Input: part model. Units: mm. Frame: model coordinates. A direction names the side the tool comes from. Give positions to 0.01 mm unless a question says otherwise; leave off trailing zeros. Loops run counter-clockwise (first coordinate to the right, second up) from the corner with the lowest first, then second, coordinate; pieces in that order, holes last. Notation, with made-up numbers: M -40,-14 L -29,-14 A24 ccw -29,10 Z; hole C 6.5,60 d11. An arc over 180 degrees is marked long. Use CSV: the item, a comma, the result in double quotes. Start each with the question number.
Q1. Reachability of faces 4 (the cylindrical face through (10.994, -24.204, 18.559)), 5 (the flat face through (4, 21.5, 0)) from +Z, -Z, +X, -X, +Y, -Y: full face, straight path, thin tool, end or side. Return the list, or none.
Q2. Section C-C, the plane x = -2.5. Output: boundary loops of the cut face in (y, z).
Q3. Pin query (flat end, axial travel): pin 1 (8 mm diameter, centred on y = -35, z = -61, fed in from +X); pin 2 (8 mm diameter, centred on x = 9, z = -45, fed in from -Y); pin 3 (4 mm diameter, centred on y = 40.5, z = 16.5, fed in from -X). Return the tip coordinate at first contact, or that it passes through.
Q4. Section A-A, the plane z = 0. Output: boundary loops of the cut face in (x, y), plus the area to 3 significant figures.
Q5. Material intervals for line 1 along Z through (x, y) = (-3, 0); line 2 along X through (y, z) = (37, 78.5); line 3 along X through (y, z) = (-57, 47), sorted ascending.
Q6. Section B-B, the plane y = 0. Output: boundary loops of the cut face in (x, z).
Q7. Pull-direction query (Y, two-part tool) for faces 1 (the cylindrical face through (5.463, -17.485, 0.713)), 2 (the flat face through (-13.6, -7.4, -16.2)), 3 (the conical face through (23, 20.87, -6.57)); classes: released by +Y, released by -Y, zero draft, split by the parting line, or undercut.
Autodesk Inventor part; units mm, degrees
ref_plane "YZ Plane" through (0, 0, 0) normal (1, 0, 0) x (0, 1, 0)
ref_plane "XZ Plane" through (0, 0, 0) normal (0, 1, 0) x (-1, 0, 0)
ref_plane "XY Plane" through (0, 0, 0) normal (0, 0, 1) x (1, 0, 0)
sketch "Sketch1" plane through (0, 0, 0) normal (0, 0, 1) x (1, 0, 0)
  line L0 (0, 87.5) -> (8, 87.5)
  line L1 (24, 0) -> (24, 17.5)
  line L2 (8, 87.5) -> (24, 17.5)
  line L3 (16, 0) -> (16, 17.5)
  line L4 (16, 17.5) -> (0, 87.5)
  line L5 (16, 0) -> (24, 0)
  point P0 (0, 0)
  dimension "d0" = 87.5
  dimension "d1" = 8
  dimension "d3" = 17.5
  dimension "d7" = 8
  dimension "d8" = 167.125
  dimension "d9" = 175
  dimension "d10" = 24
revolve "Revolution1" add sketch "Sketch1" angle 360 about axis through (16, 0, 0) along (1, 0, 0)
sketch "Sketch2" plane through (0, 0, 0) normal (0, 0, 1) x (1, 0, 0)
  line L0 (16, 0) -> (16, 24.5)
  line L1 (16, -17.5) -> (16, 17.5)
  line L2 (14.4, 24.5) -> (16, 24.5)
  line L3 (14.4, 24.5) -> (-13.6, 24.5)
  line L4 (-13.6, 24.5) -> (-13.6, 0)
  line L5 (-13.6, 0) -> (16, 0)
  point P0 (0, 0)
  dimension "d13" = 24.5
  dimension "d15" = 28
revolve "Revolution2" add sketch "Sketch2" angle 360 about axis through (-13.6, 0, 0) along (1, 0, 0)
sketch "Sketch3" plane through (0, 0, 0) normal (0, 0, 1) x (1, 0, 0)
  line L0 (14.4, 0) -> (14.4, 30.5)
  line L1 (14.4, 30.5) -> (13.0159, 30.5)
  line L2 (13.0159, 30.5) -> (9.0159, 30.5)
  line L3 (9.0159, 30.5) -> (9.0159, 0)
  line L4 (9.0159, 0) -> (14.4, 0)
  point P0 (0, 0)
  dimension "d17" = 30.5
  dimension "d18" = 4
revolve "Revolution3" add sketch "Sketch3" angle 360 about axis through (9.0159, 0, 0) along (1, 0, 0)
sketch "Sketch4" plane through (24, 0, 0) normal (1, 0, 0) x (0, 0, -1)
  circle A0 centre (0, 0) radius 17.5
extrude "Extrusion1" cut sketch "Sketch4" against normal through all
sketch "Sketch5" plane through (-13.6, 0, 0) normal (-1, 0, 0) x (0, 0, 1)
  circle A0 centre (0, 0) radius 17.5
  line L0 (0, 21.5) -> (4, 21.5)
  line L1 (0, 21.5) -> (-4, 21.5)
  line L2 (-4, 21.5) -> (-4, 17.0367)
  line L3 (4, 21.5) -> (4, 17.0367)
  line L4 (-4, 17.0367) -> (4, 17.0367)
  dimension "d23" = 4
  dimension "d24" = 4
extrude "Extrusion2" cut sketch "Sketch5" against normal through all contours A0 L2 L1 L0 L3
properties part number "Nivelador de Correia"
A:
1,face 4,"-X"
1,face 5,"+X, -X"
2,outline,"C 0,0 d49; hole M 17.04,-4 L 21.5,-4 L 21.5,4 L 17.04,4 A17.5 ccw long Z"
3,pin 1,"x = 12.84"
3,pin 2,"y = -77.23"
3,pin 3,"x = 9.55"
4,outline,"M -13.6,-24.5 L 9.02,-24.5 L 9.02,-30.5 L 13.03,-30.5 L 0,-87.5 L 8,-87.5 L 24,-17.5 L -13.6,-17.5 Z; M -13.6,21.5 L 23.09,21.5 L 8,87.5 L 0,87.5 L 13.03,30.5 L 9.02,30.5 L 9.02,24.5 L -13.6,24.5 Z"
4,area,"1,430 mm^2"
5,line 1,"-24.5 to -17.5, 17.5 to 24.5"
5,line 2,"0.16 to 8.16"
5,line 3,"3.11 to 11.11"
6,outline,"M -13.6,-24.5 L 9.02,-24.5 L 9.02,-30.5 L 13.03,-30.5 L 0,-87.5 L 8,-87.5 L 24,-17.5 L -13.6,-17.5 Z; M -13.6,17.5 L 24,17.5 L 8,87.5 L 0,87.5 L 13.03,30.5 L 9.02,30.5 L 9.02,24.5 L -13.6,24.5 Z"
7,face 1,"undercut"
7,face 2,"zero draft"
7,face 3,"split by the parting line"
